```python
from build123d import *

# Parameters (mm, degrees)
BOSS_EXTRUDE1_DEPTH                              = 19.05
F_1_4_20_TAPPED_HOLE1_D                          = 5.1054
F_1_4_20_TAPPED_HOLE1_DEPTH                      = 19.05
F_1_4_20_TAPPED_HOLE1_TIP                        = 1.533816902
SKETCH4_R                                        = 63.5
CUT_EXTRUDE1_DEPTH                               = 19.05
CSK_FOR_1_2_FLAT_HEAD_MACHINE_SCREW1_D           = 13.49248
CSK_FOR_1_2_FLAT_HEAD_MACHINE_SCREW1_CSINK_D     = 22.225
CSK_FOR_1_2_FLAT_HEAD_MACHINE_SCREW1_CSINK_ANGLE = 82
FILLET1_R                                        = 2.54
LPATTERN1_COUNT                                  = 4
LPATTERN1_PITCH                                  = 15.24


with BuildPart() as part:
    # Sketch1 → Boss-Extrude1 (new, symmetric)
    with BuildSketch(Plane(origin=(0, 0, 0), x_dir=(1, 0, 0), z_dir=(0, 1, 0))):
        with BuildLine():
            Line((0, 0), (50.421258973, 0))
            ThreePointArc((50.421258973, 0), (82.55, 12.7), (114.678741027, 0))
            Line((114.678741027, 0), (177.8, 0))
            Line((177.8, 0), (177.8, 36.59121265))
            ThreePointArc((177.8, 36.59121265), (174.397045256, 49.29121265), (165.1, 58.588257906))
            Line((165.1, 58.588257906), (101.6, 95.25))
            Line((101.6, 95.25), (101.6, 58.42))
            Line((101.6, 58.42), (76.2, 58.42))
            Line((76.2, 58.42), (76.2, 78.74))
            ThreePointArc((76.2, 78.74), (60.325, 94.615), (44.45, 78.74))
            Line((44.45, 78.74), (44.45, 66.04))
            Line((44.45, 66.04), (0, 66.04))
            Line((0, 66.04), (0, 0))
        make_face()
    extrude(amount=BOSS_EXTRUDE1_DEPTH, both=True)

    # 1/4-20 Tapped Hole1
    with Locations(Plane(origin=(66.644459855, 0, -115.431590512), x_dir=(-0.86602540378444, 0, -0.49999999999999784), z_dir=(0.49999999999999784, 0, -0.86602540378444))):
        with Locations((-66.04, 0)):
            Hole(F_1_4_20_TAPPED_HOLE1_D / 2, depth=F_1_4_20_TAPPED_HOLE1_DEPTH)
            with Locations((0, 0, -(F_1_4_20_TAPPED_HOLE1_DEPTH + F_1_4_20_TAPPED_HOLE1_TIP / 2))):  # 118° drill point
                Cone(0, F_1_4_20_TAPPED_HOLE1_D / 2, F_1_4_20_TAPPED_HOLE1_TIP, mode=Mode.SUBTRACT)

    # Sketch4 → Cut-Extrude1 (cut)
    with BuildSketch(Plane(origin=(0, 19.05, 0), x_dir=(1, 0, 0), z_dir=(0, 1, 0))):
        with Locations((82.55, -34.29)):
            Circle(SKETCH4_R)
    extrude(amount=-CUT_EXTRUDE1_DEPTH, mode=Mode.SUBTRACT)

    # CSK for 1/2 Flat Head Machine Screw1 (through all)
    with Locations(Plane(origin=(0, 19.05, 0), x_dir=(1, 0, 0), z_dir=(0, 1, 0))):
        with Locations((60.325, 78.74), (31.75, 31.75), (158.75, 31.75)):
            CounterSinkHole(CSK_FOR_1_2_FLAT_HEAD_MACHINE_SCREW1_D / 2, CSK_FOR_1_2_FLAT_HEAD_MACHINE_SCREW1_CSINK_D / 2, counter_sink_angle=CSK_FOR_1_2_FLAT_HEAD_MACHINE_SCREW1_CSINK_ANGLE)

    # Fillet1
    fillet1_edges = [part.edges().sort_by_distance(p)[0] for p in [
        (101.6, 0, -95.25),
    ]]
    fillet(fillet1_edges, radius=FILLET1_R)

    # Sketch8 → Cut-Revolve1 (revolve, cut)
    with BuildSketch(Plane(origin=(7.62, 0, 0), x_dir=(0, 0, -1), z_dir=(1, 0, 0)), mode=Mode.PRIVATE) as cut_revolve1_sk:
        Polygon((3.81, 19.05), (5.08, 17.78), (5.08, 10.16), (6.604, 9.28011819), (6.604, 2.643567375), (8.89, 1.27), (8.89, 19.05), align=None)
    cut_revolve1 = revolve(cut_revolve1_sk.sketch.rotate(Axis((7.62, 1.27, -8.89), (0, 1, 0)), 180), axis=Axis((7.62, 1.27, -8.89), (0, 1, 0)), mode=Mode.SUBTRACT)

    # LPattern1: Cut-Revolve1 ×4
    with Locations(*[(0, 0, -i * LPATTERN1_PITCH) for i in range(1, LPATTERN1_COUNT)]):
        add(cut_revolve1, mode=Mode.SUBTRACT)

    # Sketch9 → 1/16 NPT Tapped Hole1 (revolve, cut)
    with BuildSketch(Plane(origin=(7.62, 2.54, -66.04), x_dir=(0, 1, 0), z_dir=(1, 0, 0))):
        Polygon((0, 0), (0, 63.568685027), (3.0734, 61.722), (3.0734, 6.858), (3.776858756, 6.858), (3.9679118, 0.4770882), (4.445, 0), align=None)
    revolve(axis=Axis((7.62, 2.54, -72.39), (0, 0, 1)), mode=Mode.SUBTRACT)


solid = part.part
```
The listing builds one solid part. Answer for the finished solid, in the listing's coordinates (mm). A direction names the side the tool comes from. Give positions to 0.01 mm unless a question says otherwise; leave off trailing zeros. Loops run counter-clockwise (first coordinate to the right, second up) from the corner with the lowest first, then second, coordinate; pieces in that order, holes last. Notation, with made-up numbers: (34, 58) - (51, 58) arc R8 cw to (51, 68) - close; hole circle Ø2 at (68, 53.5). An arc over 180 degrees is marked (long way). Return JSON: item names as keys, results as strings. Group by question number.
1. Find section A-A (z = -31.75). Write down the section's boundary in (x, y), then the cut area to 3 significant figures.
2. Determine the mould class of faces 6 (the conical face through (11.057, 4.327, -62.417)), 7 (the cylindrical face through (3.842, 13.917, -8.394)), 8 (the conical face through (164.272, 14.271, -27.516)) for opening direction Y: pulls with the +Y half, pulls with the -Y half, needs draft (parallel to the pull), parting line crosses it, or undercut.
3. Given pin 1 Ø12 at (x, z) = (60.325, -78.74) entering from -Y; pin 2 Ø3 at (x, y) = (86.5, -0.5) entering from +Z; pin 3 Ø12.5 at (x, y) = (92.5, -9) entering from -Z; pin 4 Ø21.5 at (x, z) = (158.75, -31.75) entering from +Y, each flat-ended and moving along its own axis, determine where each tip first touches the part or whether it passes through.
4. Straight lines are drawn through the part: line 1 (X direction, y = -10, z = -78.5); line 2 (X direction, y = 14, z = -11.5); line 3 (X direction, y = 2.54, z = -31.5). For each, find the intervals that lie inside material, in ascending order. Write a range as [from, to].
5. Which of the six approach directions +Z, -Z, +X, -X, +Y, -Y give full straight-line access (tool end or side, diameter ignored) to faces 1 (the cylindrical face through (7.519, 7.425, -21.846)), 2 (the flat face through (76.2, 0, -68)), 3 (the flat face through (11, 2, -59.182)), 4 (the cylindrical face through (83.439, 9.658, -29.204)), 5 (the flat face through (23, 0, -66.04))?
6. Find section B-B (x = 31.75). Write down the section's boundary in (y, z).
7. Find section C-C (z = -8.89). Write down the section's boundary in (x, y).
8. Find section D-D (x = 128). Write down the section's boundary in (y, z), then the cut area to 3 significant figures.
Verdict:
{
 "1": {"outline": "(0, -19.05) - (25, -19.05) - (25, 14.03) - (20.64, 19.05) - (0, 19.05) - close; (38.5, -19.05) - (152, -19.05) - (152, 14.03) - (147.64, 19.05) - (42.86, 19.05) - (38.5, 14.03) - close; (165.5, -19.05) - (177.8, -19.05) - (177.8, 19.05) - (169.86, 19.05) - (165.5, 14.03) - close; hole circle Ø6.15 at (7.62, 2.54)", "area": "5,670 mm^2"},
 "2": {"face 6": "undercut", "face 7": "needs draft", "face 8": "pulls with the +Y half"},
 "3": {"pin 1": "passes through", "pin 2": "stops at z = -12.38", "pin 3": "stops at z = -58.42", "pin 4": "stops at y = 18.63"},
 "4": {"line 1": "x = [44.45, 53.58], [67.07, 76.2], [101.6, 130.61]", "line 2": "x = [0, 4.84], [10.4, 38.56], [126.54, 177.8]", "line 3": "x = [0, 4.55], [10.69, 25.01], [38.49, 152.01], [165.49, 177.8]"},
 "5": {"face 1": "+Y", "face 2": "-Z, +Y, -Y", "face 3": "-Z", "face 4": "+Z, +Y", "face 5": "-Z, -X, +Y, -Y"},
 "6": {"outline": "(-19.05, -66.04) - (19.05, -66.04) - (19.05, -42.86) - (14.03, -38.5) - (-19.05, -38.5) - close; (-19.05, -25) - (14.03, -25) - (19.05, -20.64) - (19.05, -3.81) - (0, -3.81) - (0, 0) - (-19.05, 0) - close"},
 "7": {"outline": "(0, -19.05) - (64.01, -19.05) - (64.01, 0) - (35.99, 0) - (35.99, 19.05) - (12.7, 19.05) - (11.43, 17.78) - (11.43, 10.16) - (9.91, 9.28) - (9.91, 4.59) arc R3.07 cw (long way) to (5.33, 4.59) - (5.33, 9.28) - (3.81, 10.16) - (3.81, 17.78) - (2.54, 19.05) - (0, 19.05) - close; (101.09, -19.05) - (177.8, -19.05) - (177.8, 19.05) - (129.11, 19.05) - (129.11, 0) - (101.09, 0) - close"},
 "8": {"outline": "(-19.05, -80.01) - (19.05, -80.01) - (19.05, -10.06) - (0, -10.06) - (0, 0) - (-19.05, 0) - close", "area": "2,860 mm^2"}
}
